Answer from the drawing. Dimensions are ordinates in mm from the lowest x, y and z of the part. A direction names the side the tool comes from. Coordinates: 2 decimals unless noted, no trailing zeros. Write each loop counter-clockwise with the first axis right and the second up, starting at its lowest first coordinate (ties: lowest second). Pieces come first, ordered by that corner, then holes. Notation, with made-up numbers: (-36.5, 21.5) -> (3.5, 21.5) arc R11 cw to (3.5, 37.5) -> close; hole circle Ø10 at (5, 89.5). An arc over 180 degrees is marked (long way). Answer as a JSON object with one key per item and string values. Group by question number.
(1) Flat-ended cylindrical pins translate along their axes: P1, Ø1.5, axis at y = 17.5, z = 15.5, coming from the -X side; P2, Ø10, axis at y = 5, z = 11, coming from the +X side; P3, Ø5, axis at x = 10.5, z = 11.5, coming from the +Y side. Find the tip coordinate at first contact, or state that the pin passes through.
(2) Find section C-C (z = 16). Give the vertices of the cut face in (x, y), then the cut area to 3 significant figures.
(3) Find section B-B (x = 13.5). Give the vertices of the cut face in (y, z).
(4) Find section D-D (y = 9.5). Give the vertices of the cut face in (x, z), then the cut area to 3 significant figures.
(5) For a pull along X with two mould halves and no side action, classify the marked faces 1, 2 and 3 as +X half, -X half, draft (parallel to the pull), parting line (faces both ways), or undercut.
(6) Find section A-A (y = 13.5). Give the vertices of the cut face in (x, z).
(7) Which of the six approach directions +Z, -Z, +X, -X, +Y, -Y give full straight-line access (tool end or side, diameter ignored) to the marked faces 4, 5 and 6?
(8) Straight lines are drawn through the part: L1, parallel to Z at x = 16.5, y = 25.25; L2, parallel to Z at x = 23.75, y = 10.5; L3, parallel to X at y = 13.75, z = 22. For each, find the intervals that lie inside material, in ascending order.
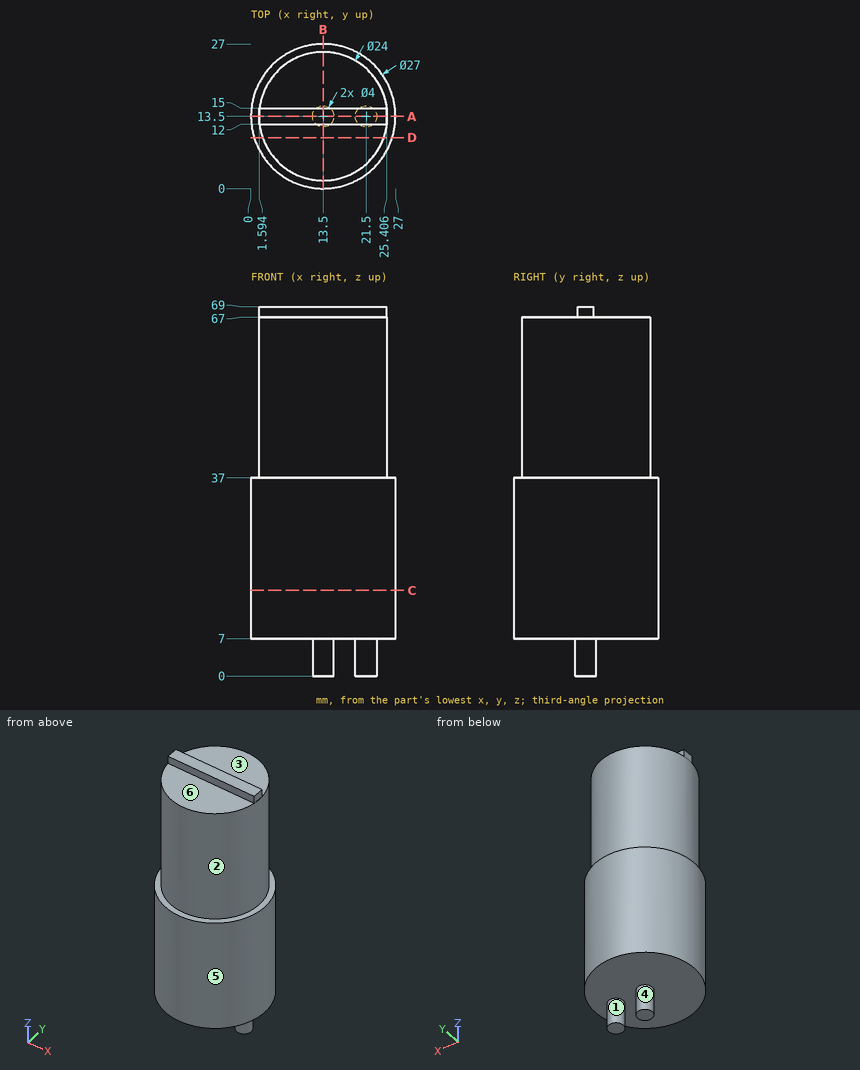
Results below:
{
 "1": {"P1": "stops at x = 0.4", "P2": "stops at x = 26.54", "P3": "stops at y = 26.99"},
 "2": {"outline": "circle Ø27 at (13.5, 13.5)", "area": "573 mm2"},
 "3": {"outline": "(0, 7) -> (11.5, 7) -> (11.5, 0) -> (15.5, 0) -> (15.5, 7) -> (27, 7) -> (27, 37) -> (25.5, 37) -> (25.5, 67) -> (15, 67) -> (15, 69) -> (12, 69) -> (12, 67) -> (1.5, 67) -> (1.5, 37) -> (0, 37) -> close"},
 "4": {"outline": "(0.61, 7) -> (26.39, 7) -> (26.39, 37) -> (24.81, 37) -> (24.81, 67) -> (2.19, 67) -> (2.19, 37) -> (0.61, 37) -> close", "area": "1,450 mm2"},
 "5": {"face 1": "undercut", "face 2": "parting line", "face 3": "draft"},
 "6": {"outline": "(0, 7) -> (11.5, 7) -> (11.5, 0) -> (15.5, 0) -> (15.5, 7) -> (19.5, 7) -> (19.5, 0) -> (23.5, 0) -> (23.5, 7) -> (27, 7) -> (27, 37) -> (25.5, 37) -> (25.5, 67) -> (25.41, 67) -> (25.41, 69) -> (1.59, 69) -> (1.59, 67) -> (1.5, 67) -> (1.5, 37) -> (0, 37) -> close"},
 "7": {"face 4": "-Z", "face 5": "+Z, -Z", "face 6": "+Z, +X, -X, -Y"},
 "8": {"L1": "z = 7 to 37", "L2": "z = 7 to 67", "L3": "x = 0 to 27"}
}
